Could you check a few things on this model? Use its own coordinates, in mm. Face numbers are marked on the shaded views. A direction names the side the tool comes from. Coordinates: 2 decimals unless noted, no trailing zeros. Order: outer loops, then holes, each group sorted by start corner. A loop starts at its lowest first (then second) coordinate and runs counter-clockwise, first axis right, second up. Notation, with made-up numbers: (-36, -19.75) - (4, -19.75) arc R19 ccw to (4, -3.75) - close; hole circle Ø2 at (12, 43). An arc over 180 degrees is marked (long way). Answer as a JSON object with one key per item and string values. Group by question number.
(1) Please list where these lines run through material, in increasing order: probe 1 along Z at (x, y) = (445.5, 50.8); probe 2 along Y at (x, z) = (-446, 82.55); probe 3 along X at (y, z) = (96, -46.5).
(2) Imagine slicing it at A-A, the plane y = 50.8. Write out the boundary of the cut face in (x, z).
(3) Imagine slicing it at B-B, the plane z = 0. Write out the boundary of the cut face in (x, y).
(4) Imagine slicing it at D-D, the plane z = -82.55. Write out the boundary of the cut face in (x, y).
(5) Which directions (+Z, -Z, +X, -X, +Y, -Y) give clear straight access to the entire face, cutting with the end or side of a thin tool? Please do the marked faces 3 and 4.
(6) Imagine slicing it at C-C, the plane x = 270.5. Write out the boundary of the cut face in (y, z) (3 decimals).
(7) Will this pin go through, and if not, where does the flat tip stop? P1, Ø23, axis at y = 50.8, z = 82.55, coming from the -X side.
(8) We'd pull the mould along Z, two halves only. Please class the marked faces 1 and 2: pulls with the +Z half, pulls with the -Z half, needs draft (parallel to the pull), parting line crosses it, or undercut.
from build123d import *

# Parameters (mm, degrees)
SKETCH1_W               = 914.4
SKETCH1_H               = 215.9
BOSS_EXTRUDE1_DEPTH     = 101.6
CUT_EXTRUDE1_REACH      = 482.633
SKETCH2_W               = 838.2
SKETCH2_H               = 120.65
CUT_EXTRUDE2_DEPTH      = 516.720088808
CUT_EXTRUDE2_DEPTH_BACK = 516.720088808
SKETCH3_W               = 838.2
SKETCH3_H               = 63.5
CUT_EXTRUDE3_DEPTH      = 927.33855717
CUT_EXTRUDE3_DEPTH_BACK = 927.33855717
SKETCH4_R               = 12.7
CUT_EXTRUDE4_REACH      = 928.339
SKETCH5_R               = 19.05


with BuildPart() as part:
    # Sketch1 → Boss-Extrude1 (new body)
    with BuildSketch(Plane(origin=(0, 0, 0), x_dir=(1, 0, 0), z_dir=(0, 1, 0))):
        Rectangle(SKETCH1_W, SKETCH1_H)
    extrude(amount=BOSS_EXTRUDE1_DEPTH)

    # Sketch2 → Cut-Extrude1 (cut, up to next)
    with BuildSketch(Plane(origin=(0, 101.6, 0), x_dir=(1, 0, 0), z_dir=(0, 1, 0)), mode=Mode.PRIVATE) as cut_extrude1_sk1:
        Rectangle(SKETCH2_W, SKETCH2_H)
    cut_extrude1_tool1 = extrude(cut_extrude1_sk1.sketch, amount=-CUT_EXTRUDE1_REACH, mode=Mode.PRIVATE) & part.part
    add(cut_extrude1_tool1.solids().sort_by_distance((0, 101.6, 0))[0], mode=Mode.SUBTRACT)

    # Sketch3 → Cut-Extrude2 (cut, two sides: drawn at the far end of the back side and taken through both)
    with BuildSketch(Plane.XY.offset(107.95).offset(-CUT_EXTRUDE2_DEPTH_BACK)):
        with Locations((0, 50.8)):
            Rectangle(SKETCH3_W, SKETCH3_H)
    extrude(amount=CUT_EXTRUDE2_DEPTH + CUT_EXTRUDE2_DEPTH_BACK, mode=Mode.SUBTRACT)

    # Sketch4 → Cut-Extrude3 (cut, two sides: drawn at the far end of the back side and taken through both)
    with BuildSketch(Plane.ZY.offset(457.2).offset(-CUT_EXTRUDE3_DEPTH_BACK)):
        with Locations((82.55, 50.8)):
            Circle(SKETCH4_R)
        with Locations((-82.55, 50.8)):
            Circle(SKETCH4_R)
    extrude(amount=CUT_EXTRUDE3_DEPTH + CUT_EXTRUDE3_DEPTH_BACK, mode=Mode.SUBTRACT)

    # Sketch5 → Cut-Extrude4 (cut, up to next)
    with BuildSketch(Plane.ZY.offset(457.2), mode=Mode.PRIVATE) as cut_extrude4_sk1:
        with Locations((0, 50.8)):
            Circle(SKETCH5_R)
    cut_extrude4_tool1 = extrude(cut_extrude4_sk1.sketch, amount=-CUT_EXTRUDE4_REACH, mode=Mode.PRIVATE) & part.part
    add(cut_extrude4_tool1.solids().sort_by_distance((-457.2, 50.8, 0))[0], mode=Mode.SUBTRACT)


solid = part.part
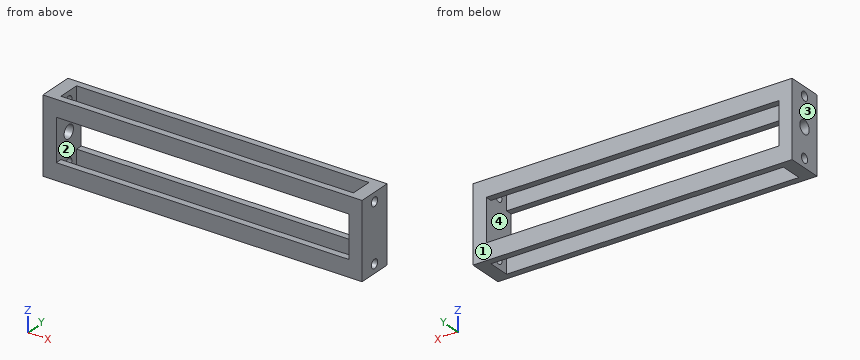
Result set:
{
 "1": {"probe 1": "z = -107.95 to -95.25, -69.85 to 69.85, 95.25 to 107.95", "probe 2": "y = 0 to 38.1, 63.5 to 101.6", "probe 3": "x = -457.2 to -419.1, 419.1 to 457.2"},
 "2": {"outline": "(-457.2, -107.95) - (-419.1, -107.95) - (-419.1, -95.25) - (-457.2, -95.25) - close; (-457.2, -69.85) - (-419.1, -69.85) - (-419.1, -19.05) - (-457.2, -19.05) - close; (-457.2, 19.05) - (-419.1, 19.05) - (-419.1, 69.85) - (-457.2, 69.85) - close; (-457.2, 95.25) - (-419.1, 95.25) - (-419.1, 107.95) - (-457.2, 107.95) - close; (419.1, -107.95) - (457.2, -107.95) - (457.2, -95.25) - (419.1, -95.25) - close; (419.1, -69.85) - (457.2, -69.85) - (457.2, 69.85) - (419.1, 69.85) - close; (419.1, 95.25) - (457.2, 95.25) - (457.2, 107.95) - (419.1, 107.95) - close"},
 "3": {"outline": "(-457.2, 0) - (-419.1, 0) - (-419.1, 31.75) - (-457.2, 31.75) - close; (-457.2, 69.85) - (-419.1, 69.85) - (-419.1, 101.6) - (-457.2, 101.6) - close; (419.1, 0) - (457.2, 0) - (457.2, 101.6) - (419.1, 101.6) - close"},
 "4": {"outline": "(-457.2, 0) - (457.2, 0) - (457.2, 38.1) - (419.1, 38.1) - (419.1, 19.05) - (-419.1, 19.05) - (-419.1, 38.1) - (-457.2, 38.1) - close; (-457.2, 63.5) - (-419.1, 63.5) - (-419.1, 82.55) - (419.1, 82.55) - (419.1, 63.5) - (457.2, 63.5) - (457.2, 101.6) - (-457.2, 101.6) - close"},
 "5": {"face 3": "+Z, -Z, -X, +Y, -Y", "face 4": "none"},
 "6": {"outline": "(0, -107.95) - (19.05, -107.95) - (19.05, -60.325) - (0, -60.325) - close; (0, 60.325) - (19.05, 60.325) - (19.05, 107.95) - (0, 107.95) - close; (82.55, -107.95) - (101.6, -107.95) - (101.6, -60.325) - (82.55, -60.325) - close; (82.55, 60.325) - (101.6, 60.325) - (101.6, 107.95) - (82.55, 107.95) - close"},
 "7": {"P1": "passes through"},
 "8": {"face 1": "needs draft", "face 2": "undercut"}
}
